Here's how the part is built. I have some questions about the finished solid (model axes, mm). Coordinates: 2 decimals unless noted, no trailing zeros. Loops run counter-clockwise (first coordinate to the right, second up) from the corner with the lowest first, then second, coordinate; pieces in that order, holes last. Notation, with made-up numbers: M -5,15.25 L 38,15.25 A28 cw 38,35.25 Z; hole C -27.5,21.5 d3. An arc over 180 degrees is marked long. Use CSV: the item, a comma, the result in double quotes. Start each with the question number.
Q1. If we section it at D-D (x = -3.5): Please give me the cut outline in (y, z), and give its area (3 significant figures).
Q2. Please list where these lines run through material, in increasing order: probe 1 along X at (y, z) = (-12, 2.55); probe 2 along X at (y, z) = (16.5, 4.35); probe 3 along Y at (x, z) = (0, 0.8). Write a range as [from, to].
Q3. If we section it at C-C (z = 2.9): State how many separate pieces and enclosed holes the cut face has, and give its area (3 significant figures).
Q4. If we section it at A-A (y = -27.5): Please give me the cut outline in (x, z).
Q5. If we section it at B-B (y = 22.5): Please give me the cut outline in (x, z), and give its area (3 significant figures).
Q6. For pin 1 Ø1.2 at (y, z) = (-33, 2.5) entering from -X; pin 2 Ø0.6 at (x, z) = (-24, 3) entering from -Y; pin 3 Ø2.5 at (y, z) = (-26.5, 2.5) entering from +X, each with a flat end and sliding along its axis, tell me the tip position at first contact or that it passes through.
from build123d import *
from OCP.BRepFilletAPI import BRepFilletAPI_MakeChamfer

# Parameters (mm, degrees)
SKETCH1_W           = 1.5
SKETCH1_H           = 4
BOSS_EXTRUDE2_DEPTH = 5
FILLET1_R           = 0.5
CHAMFER1_SIZE       = 0.3
CHAMFER1_SIZE2      = 5.724341006
FILLET2_R           = 1


with BuildPart() as part:
    # Sketch1 → Boss-Extrude2 (new body)
    with BuildSketch(Plane.XY):
        with BuildLine():
            Line((-23, 0), (-23, -38))
            Line((-23, -38), (-18, -38))
            Line((-18, -38), (-18, 0))
            Line((-18, 0), (-19, 0))
            ThreePointArc((-19, 0), (-20.184067393, 2.97246837), (-22, 5.606851138))
            ThreePointArc((-22, 5.606851138), (-24.550960709, 9.359484468), (-26.147686675, 13.606851138))
            ThreePointArc((-26.147686675, 13.606851138), (-30.048729273, 58.796026105), (-20, 103.026136974))
            ThreePointArc((-20, 103.026136974), (-16.753739062, 108.568721435), (-12, 112.888491974))
            ThreePointArc((-12, 112.888491974), (-8.655764836, 114.460632304), (-5, 115))
            Line((-5, 115), (0, 115))
            Line((0, 115), (5, 115))
            ThreePointArc((5, 115), (8.655764836, 114.460632304), (12, 112.888491974))
            ThreePointArc((12, 112.888491974), (16.753739062, 108.568721435), (20, 103.026136974))
            ThreePointArc((20, 103.026136974), (30.048729273, 58.796026105), (26.147686675, 13.606851138))
            ThreePointArc((26.147686675, 13.606851138), (24.550960709, 9.359484468), (22, 5.606851138))
            ThreePointArc((22, 5.606851138), (20.184067393, 2.97246837), (19, 0))
            Line((19, 0), (18, 0))
            Line((18, 0), (18, -38))
            Line((18, -38), (23, -38))
            Line((23, -38), (23, 0))
            Line((23, 0), (25, 0))
            ThreePointArc((25, 0), (25.153863701, 1.240298929), (25.773026769, 2.325956595))
            ThreePointArc((25.773026769, 2.325956595), (28.989837998, 7.058100445), (31.003340596, 12.414112692))
            ThreePointArc((31.003340596, 12.414112692), (35.036954168, 59.138972746), (24.646734179, 104.872176375))
            ThreePointArc((24.646734179, 104.872176375), (20.63684435, 111.718561641), (14.764867241, 117.05448635))
            ThreePointArc((14.764867241, 117.05448635), (10.08229677, 119.521890335), (5, 121))
            Line((5, 121), (-5, 121))
            ThreePointArc((-5, 121), (-10.08229677, 119.521890335), (-14.764867241, 117.05448635))
            ThreePointArc((-14.764867241, 117.05448635), (-20.63684435, 111.718561641), (-24.646734179, 104.872176375))
            ThreePointArc((-24.646734179, 104.872176375), (-35.036954168, 59.138972746), (-31.003340596, 12.414112692))
            ThreePointArc((-31.003340596, 12.414112692), (-28.989837998, 7.058100445), (-25.773026769, 2.325956595))
            ThreePointArc((-25.773026769, 2.325956595), (-25.153863701, 1.240298929), (-25, 0))
            Line((-25, 0), (-23, 0))
        make_face()
        with Locations((-20.5, -33)):
            Rectangle(SKETCH1_W, SKETCH1_H, mode=Mode.SUBTRACT)
        with Locations((20.5, -33)):
            Rectangle(SKETCH1_W, SKETCH1_H, mode=Mode.SUBTRACT)
    extrude(amount=BOSS_EXTRUDE2_DEPTH)

    # Fillet1
    fillet1_edges = [part.edges().sort_by_distance(p)[0] for p in [
        (-25, 0, 2.5),
        (25, 0, 2.5),
        (18, 0, 2.5),
        (19, 0, 2.5),
        (-19, 0, 2.5),
        (-18, 0, 2.5),
    ]]
    fillet(fillet1_edges, radius=FILLET1_R)

    # Chamfer1: one chamfer whose edges measure the first distance from different faces: ONE call of the kernel's chamfer builder (chamfer() names one face for all edges)
    chamfer1_edges_1 = [part.edges().sort_by_distance(p)[0] for p in [
        (-23, 0, 2.5),
    ]]
    chamfer1_side_1 = [part.faces().sort_by_distance(p)[0] for p in [
        (-23.750387455, 0, 2.5),
    ]]
    chamfer1_edges_2 = [part.edges().sort_by_distance(p)[0] for p in [
        (23, 0, 2.5),
    ]]
    chamfer1_side_2 = [part.faces().sort_by_distance(p)[0] for p in [
        (23.750387455, 0, 2.5),
    ]]
    chamfer1 = BRepFilletAPI_MakeChamfer(part.part.solid().wrapped)
    for e in chamfer1_edges_1:
        chamfer1.Add(CHAMFER1_SIZE, CHAMFER1_SIZE2, e.wrapped, chamfer1_side_1[0].wrapped)  # the first distance lies on this face
    for e in chamfer1_edges_2:
        chamfer1.Add(CHAMFER1_SIZE, CHAMFER1_SIZE2, e.wrapped, chamfer1_side_2[0].wrapped)  # the first distance lies on this face
    add(Compound.cast(chamfer1.Shape()), mode=Mode.REPLACE)

    # Fillet2
    fillet2_edges = [part.edges().sort_by_distance(p)[0] for p in [
        (-18, -38, 2.5),
        (-23, -38, 2.5),
        (23, -38, 2.5),
        (18, -38, 2.5),
    ]]
    fillet(fillet2_edges, radius=FILLET2_R)


solid = part.part
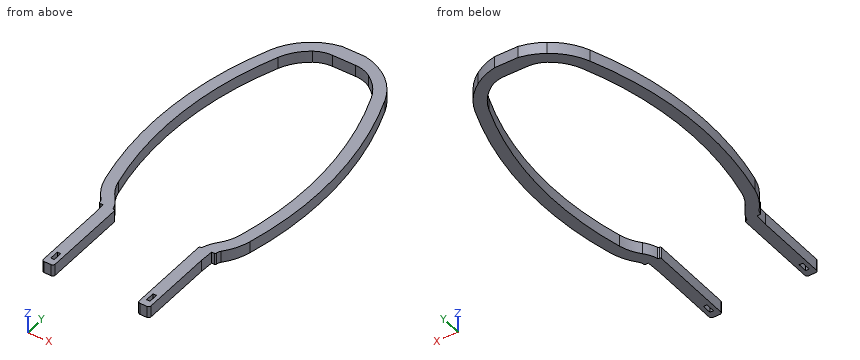
Results below:
1,outline,"M 115,0 L 121,0 L 121,5 L 115,5 Z"
1,area,"30.0 mm^2"
2,probe 1,"[-23, -18], [18, 23]"
2,probe 2,"[-31.95, -26.83], [26.83, 31.95]"
2,probe 3,"[115, 121]"
3,separate pieces,"1"
3,enclosed holes,"2"
3,area,"1,740 mm^2"
4,outline,"M -23,0 L -18,0 L -18,5 L -23,5 Z; M 18,0 L 23,0 L 23,5 L 18,5 Z"
5,outline,"M -33.12,0 L -28.04,0 L -28.04,5 L -33.12,5 Z; M 28.04,0 L 33.12,0 L 33.12,5 L 28.04,5 Z"
5,area,"50.8 mm^2"
6,pin 1,"x = -23"
6,pin 2,"y = 0"
6,pin 3,"x = 23"
